```python
from build123d import *

# Parameters (mm, degrees)
BOSS_EXTRUDE1_DEPTH     = 10
SKETCH2_R               = 10
BOSS_EXTRUDE2_DEPTH     = 1200
SKETCH4_W               = 50
SKETCH4_H               = 50
BOSS_EXTRUDE3_DEPTH     = 860
CUT_EXTRUDE2_DEPTH      = 1468.122841414
CUT_EXTRUDE2_DEPTH_BACK = 1468.122841414
SKETCH6_R               = 15


with BuildPart() as part:
    # Sketch1 → Boss-Extrude1 (new, symmetric)
    with BuildSketch(Plane(origin=(0, 0, 0), x_dir=(0, 0, -1), z_dir=(1, 0, 0))):
        with BuildLine():
            Line((150, -20), (-150, -20))
            ThreePointArc((-150, -20), (-170, 0), (-150, 20))
            Line((-150, 20), (150, 20))
            ThreePointArc((150, 20), (170, 0), (150, -20))
        make_face()
        with BuildLine():
            Line((-150, 15), (150, 15))
            ThreePointArc((150, 15), (165, 0), (150, -15))
            Line((150, -15), (-150, -15))
            ThreePointArc((-150, -15), (-165, 0), (-150, 15))
        make_face(mode=Mode.SUBTRACT)
    boss_extrude1 = extrude(amount=BOSS_EXTRUDE1_DEPTH, both=True)

    # Sketch2 → Boss-Extrude2 (add)
    with BuildSketch(Plane.XZ.offset(20)):
        with Locations(Location((0, 0, 0), (0, 0, 180))):
            Circle(SKETCH2_R)
    boss_extrude2 = extrude(amount=BOSS_EXTRUDE2_DEPTH)

    # Sketch4 → Boss-Extrude3 (add)
    with BuildSketch(Plane(origin=(0, 0, 0), x_dir=(0, 0, -1), z_dir=(1, 0, 0))):
        with Locations((0, -1181.413801262)):
            Rectangle(SKETCH4_W, SKETCH4_H)
    extrude(amount=-BOSS_EXTRUDE3_DEPTH)

    # Sketch6 → Cut-Extrude2 (cut, two sides: drawn at the far end of the back side and taken through both)
    with BuildSketch(Plane(origin=(0, -1156.413801262, 0), x_dir=(1, 0, 0), z_dir=(0, 1, 0)).offset(-CUT_EXTRUDE2_DEPTH_BACK)):
        with Locations(Location((-645, 0, 0), (0, 0, 270))):
            Circle(SKETCH6_R)
        with Locations(Location((-430, 0, 0), (0, 0, 270))):
            Circle(SKETCH6_R)
        with Locations(Location((-215, 0, 0), (0, 0, 270))):
            Circle(SKETCH6_R)
    extrude(amount=CUT_EXTRUDE2_DEPTH + CUT_EXTRUDE2_DEPTH_BACK, mode=Mode.SUBTRACT)

    # Mirror1: Boss-Extrude2 across plane
    add(boss_extrude2.mirror(Plane(origin=(-430, 0, 0), x_dir=(0, 0, 1), z_dir=(1, 0, 0))))

    # Mirror2: Boss-Extrude1 across plane
    add(boss_extrude1.mirror(Plane(origin=(-430, 0, 0), x_dir=(0, 0, 1), z_dir=(1, 0, 0))))


solid = part.part
```
Source: CAD feature listing. Evaluate the final solid. Frame: model axes, mm. A direction names the side the tool comes from. Round coordinates to 2 decimals unless told otherwise and drop trailing zeros. Order: outer loops, then holes, each group sorted by start corner. A loop starts at its lowest first (then second) coordinate and runs counter-clockwise, first axis right, second up. Notation, with made-up numbers: (56, 66) -> (114, 66) arc R18 ccw to (114, 78) -> close; hole circle Ø4 at (35.5, -4.5). An arc over 180 degrees is marked (long way). One line per item, written item: value. Start each with the question number.
Q1. Section query D-D (x = -750). Return the cut outline in (y, z).
Q2. Material intervals for probe 1 along X at (y, z) = (-1185, 0); probe 2 along Z at (x, y) = (-645, -1176); probe 3 along Y at (x, z) = (-382, 16.5), sorted ascending.
Q3. Section query A-A (y = 0). Return the cut outline in (x, z), plus the area to 3 significant figures.
Q4. Access query for faces 5 (the cylindrical face through (-229.643, -1181.764, -3.252)), 6 (the flat face through (-10, 16, -13)). Directions: +Z, -Z, +X, -X, +Y, -Y. A direction counts if a zero-diameter tool reaches every point of the face in a straight line with its end or side. Return the directions, or none.
Q5. Section query B-B (z = 76.5). Return the cut outline in (x, y).
Q6. Section query C-C (y = -144). Return the cut outline in (x, z).
Q7. Pin query (flat end, axial travel): pin 1 (10 mm diameter, centred on x = -860.5, z = -76.5, fed in from -Y); pin 2 (7.5 mm diameter, centred on y = -1188.5, z = -15.5, fed in from -X); pin 3 (25 mm diameter, centred on x = -596.5, y = -1174, fed in from +Z). Return the tip coordinate at first contact, or that it passes through.
Q8. Draft query along X for faces 1 (the flat face through (10, 16, -13)), 2 (the flat face through (-424, -1206.414, 17)), 3 (the flat face through (-424, -1182, 25)), 4 (the flat face through (-870, 16, -13)). Return one class per face: pulls with the +X half, pulls with the -X half, needs draft (parallel to the pull), parting line crosses it, or undercut.
Findings below:
1. outline: (-1206.41, -25) -> (-1156.41, -25) -> (-1156.41, 25) -> (-1206.41, 25) -> close
2. probe 1: -870 to -660, -630 to -445, -415 to -230, -200 to 10
2. probe 2: -25 to -15, 15 to 25
2. probe 3: -1206.41 to -1156.41
3. outline: (-870, -170) -> (-850, -170) -> (-850, -165) -> (-870, -165) -> close; (-870, 165) -> (-850, 165) -> (-850, 170) -> (-870, 170) -> close; (-10, -170) -> (10, -170) -> (10, -165) -> (-10, -165) -> close; (-10, 165) -> (10, 165) -> (10, 170) -> (-10, 170) -> close
3. area: 400 mm²
4. face 5: +Y, -Y
4. face 6: +Z, -Z, +Y
5. outline: (-870, -20) -> (-850, -20) -> (-850, -15) -> (-870, -15) -> close; (-870, 15) -> (-850, 15) -> (-850, 20) -> (-870, 20) -> close; (-10, -20) -> (10, -20) -> (10, -15) -> (-10, -15) -> close; (-10, 15) -> (10, 15) -> (10, 20) -> (-10, 20) -> close
6. outline: circle Ø20 at (-860, 0); circle Ø20 at (0, 0)
7. pin 1: y = -20
7. pin 2: x = -860
7. pin 3: z = 25
8. face 1: pulls with the +X half
8. face 2: undercut
8. face 3: needs draft
8. face 4: pulls with the -X half
